CAD build for the part. Positions are in the model's coordinates, mm. Coordinates: 2 decimals unless noted, no trailing zeros. Write each loop counter-clockwise with the first axis right and the second up, starting at its lowest first coordinate (ties: lowest second). Pieces come first, ordered by that corner, then holes. Notation, with made-up numbers: (52.5, 12.5) - (88.5, 12.5) arc R11 ccw to (88.5, 25.5) - close; hole circle Ø8 at (36, 16.25). An arc over 180 degrees is marked (long way). One line per question, with ' | ' between items. Start each with the question number.
1. Flat gauge pins, fed straight in: P1, Ø4, axis at x = -27, z = 34, coming from the -Y side; P2, Ø10, axis at y = 8.5, z = 11, coming from the -X side; P3, Ø12, axis at x = 34.5, y = 19, coming from the +Z side; P4, Ø2, axis at x = -47, z = 35, coming from the +Y side. Where does each tip first touch, or does it go through?
2. Band-saw the part on C-C, the plane y = 6. Write the cut outline in (x, z).
3. Band-saw the part on A-A, the plane z = 30. Write the cut outline in (x, y) (3 decimals).
4. Probe line 1 (Y direction, x = -2, z = 59); line 2 (X direction, y = 17, z = 38); line 3 (X direction, y = 30, z = 9.5). List the from-to ranges inside material, lowest first.
5. Two-plate mould, pull along X, no slides. Class faces 1 (the cylindrical face through (47.28, 10.85, 31.31)), 2 (the cylindrical face through (-48.33, 11.506, 31.306)), 3 (the cylindrical face through (1.25, 2.55, 31.31)), 4 (the flat face through (0, -2.54, 31)): +X half, -X half, draft (parallel to the pull), parting line (faces both ways), or undercut.
6. Band-saw the part on B-B, the plane y = 14. Write the cut outline in (x, z).
7. Band-saw the part on D-D, the plane x = 12. Write the cut outline in (y, z), then the cut area to 3 significant figures.
from build123d import *

# Parameters (mm, degrees)
SKETCH1_W           = 12.7
SKETCH1_H           = 5.08
BOSS_EXTRUDE1_DEPTH = 63.5


with BuildPart() as part:
    # Sketch1 → Boss-Extrude1 (new body)
    with BuildSketch(Plane.XY):
        Rectangle(SKETCH1_W, SKETCH1_H)
        with BuildLine():
            Line((-73.690101608, 45.085), (-78.089510659, 42.545))
            ThreePointArc((-78.089510659, 42.545), (0, -2.54), (78.089510659, 42.545))
            Line((78.089510659, 42.545), (73.690101608, 45.085))
            ThreePointArc((73.690101608, 45.085), (0, 2.54), (-73.690101608, 45.085))
        make_face()
    extrude(amount=BOSS_EXTRUDE1_DEPTH)


solid = part.part
Filled in:
1) P1: stops at y = 0.99 | P2: stops at x = -51.34 | P3: passes through | P4: stops at y = 17.37
2) outline: (-38.3, 0) - (-24.02, 0) - (-24.02, 63.5) - (-38.3, 63.5) - close; (24.02, 0) - (38.3, 0) - (38.3, 63.5) - (24.02, 63.5) - close
3) outline: (-78.09, 42.545) arc R90.17 ccw to (-6.35, -2.316) - (-6.35, -2.54) - (6.35, -2.54) - (6.35, -2.316) arc R90.17 ccw to (78.09, 42.545) - (73.69, 45.085) arc R85.09 cw to (-73.69, 45.085) - close
4) line 1: y = -2.54 to 2.56 | line 2: x = -56.05 to -47.45, 47.45 to 56.05 | line 3: x = -69.35 to -62.6, 62.6 to 69.35
5) face 1: +X half | face 2: -X half | face 3: undercut | face 4: draft
6) outline: (-52.05, 0) - (-42.65, 0) - (-42.65, 63.5) - (-52.05, 63.5) - close; (42.65, 0) - (52.05, 0) - (52.05, 63.5) - (42.65, 63.5) - close
7) outline: (-1.74, 0) - (3.39, 0) - (3.39, 63.5) - (-1.74, 63.5) - close | area: 326 mm²
